CAD build for the part. Positions are in the model's coordinates, mm. A direction names the side the tool comes from. Give positions to 0.01 mm unless a question says otherwise; leave off trailing zeros. Order: outer loops, then holes, each group sorted by start corner. A loop starts at its lowest first (then second) coordinate and runs counter-clockwise, first axis right, second up.
Item 1: Band-saw the part on A-A on x = 0. Give the cut face in (y, z), plus the area to 3 significant figures.
Item 2: Band-saw the part on D-D on x = 4.5. Give the cut face in (y, z), plus the area to 3 significant figures.
Item 3: Two-plate mould, pull along Z, no slides. Class faces 1 (the cylindrical face through (14.14, 24.65, -14.1)), 2 (the flat face through (0, 50, -4)), 3 (the flat face through (-14, 25, -3.1)), 4 (the flat face through (-13.25, 25, 11)): released by +Z, released by -Z, zero draft, split by the parting line, or undercut.
Item 4: Band-saw the part on C-C on y = 17. Count the separate pieces of the cut face and the enclosed holes in it, plus the area to 3 significant figures.
Item 5: Wall check: L1, parallel to Z at x = -11, y = 19.5; L2, parallel to X at y = 24, z = 0; L3, parallel to X at y = 19, z = -6. Give the ranges that are in metal, low to high.
Item 6: Which spindle directions (+Z, -Z, +X, -X, +Y, -Y) get a long thin tool onto all of the face, cutting with end or side? Do faces 5 (the flat face through (-9.5, 25, -12)), 6 (the flat face through (15, 25, 8)). Say none if no direction does.
Item 7: Band-saw the part on B-B on z = 0. Give the cut face in (x, y).
Item 8: Flat gauge pins, fed straight in: P1, Ø6, axis at x = 11, z = -12, coming from the -Y side; P2, Ø1, axis at y = 19.5, z = 13, coming from the -X side; P3, Ø4.5, axis at x = 0, z = 0, coming from the +Y side; P4, Ø0.8, axis at y = 31.5, z = -13, coming from the -X side. Where does each tip first touch, or does it go through?
```python
from build123d import *

# Parameters (mm, degrees)
SKETCH2_R           = 2.5
BOSS_EXTRUDE1_DEPTH = 50


with BuildPart() as part:
    # Sketch2 → Boss-Extrude1 (new body)
    with BuildSketch(Plane(origin=(0, 0, 0), x_dir=(1, 0, 0), z_dir=(0, 1, 0))):
        with BuildLine():
            Line((3.6, -15), (12, -15))
            ThreePointArc((12, -15), (14.121320344, -14.121320344), (15, -12))
            Line((15, -12), (15, -3.6))
            ThreePointArc((15, -3.6), (14.853553391, -3.246446609), (14.5, -3.1))
            Line((14.5, -3.1), (12.5, -3.1))
            ThreePointArc((12.5, -3.1), (12.146446609, -3.246446609), (12, -3.6))
            Line((12, -3.6), (12, -5.6))
            Line((12, -5.6), (12.5, -5.6))
            ThreePointArc((12.5, -5.6), (12.853553391, -5.746446609), (13, -6.1))
            Line((13, -6.1), (13, -8.25))
            Line((13, -8.25), (10.492640687, -8.25))
            ThreePointArc((10.492640687, -8.25), (9.727273822, -8.097759065), (9.078427125, -7.664213562))
            Line((9.078427125, -7.664213562), (5.25, -3.835786438))
            Line((5.25, -3.835786438), (5.25, 3.835786438))
            Line((5.25, 3.835786438), (9.078427125, 7.664213562))
            ThreePointArc((9.078427125, 7.664213562), (9.727273822, 8.097759065), (10.492640687, 8.25))
            Line((10.492640687, 8.25), (13, 8.25))
            Line((13, 8.25), (13, 6.1))
            ThreePointArc((13, 6.1), (12.853553391, 5.746446609), (12.5, 5.6))
            Line((12.5, 5.6), (12, 5.6))
            Line((12, 5.6), (12, 3.6))
            ThreePointArc((12, 3.6), (12.146446609, 3.246446609), (12.5, 3.1))
            Line((12.5, 3.1), (14.5, 3.1))
            ThreePointArc((14.5, 3.1), (14.853553391, 3.246446609), (15, 3.6))
            Line((15, 3.6), (15, 12))
            ThreePointArc((15, 12), (14.121320344, 14.121320344), (12, 15))
            Line((12, 15), (-12, 15))
            ThreePointArc((-12, 15), (-14.121320344, 14.121320344), (-15, 12))
            Line((-15, 12), (-15, 3.6))
            ThreePointArc((-15, 3.6), (-14.853553391, 3.246446609), (-14.5, 3.1))
            Line((-14.5, 3.1), (-12.5, 3.1))
            ThreePointArc((-12.5, 3.1), (-12.146446609, 3.246446609), (-12, 3.6))
            Line((-12, 3.6), (-12, 5.6))
            Line((-12, 5.6), (-12.5, 5.6))
            ThreePointArc((-12.5, 5.6), (-12.853553391, 5.746446609), (-13, 6.1))
            Line((-13, 6.1), (-13, 8.25))
            Line((-13, 8.25), (-10.492640687, 8.25))
            ThreePointArc((-10.492640687, 8.25), (-9.727273822, 8.097759065), (-9.078427125, 7.664213562))
            Line((-9.078427125, 7.664213562), (-5.25, 3.835786438))
            Line((-5.25, 3.835786438), (-5.25, -3.835786438))
            Line((-5.25, -3.835786438), (-9.078427125, -7.664213562))
            ThreePointArc((-9.078427125, -7.664213562), (-9.727273822, -8.097759065), (-10.492640687, -8.25))
            Line((-10.492640687, -8.25), (-13, -8.25))
            Line((-13, -8.25), (-13, -6.1))
            ThreePointArc((-13, -6.1), (-12.853553391, -5.746446609), (-12.5, -5.6))
            Line((-12.5, -5.6), (-12, -5.6))
            Line((-12, -5.6), (-12, -3.6))
            ThreePointArc((-12, -3.6), (-12.146446609, -3.246446609), (-12.5, -3.1))
            Line((-12.5, -3.1), (-14.5, -3.1))
            ThreePointArc((-14.5, -3.1), (-14.853553391, -3.246446609), (-15, -3.6))
            Line((-15, -3.6), (-15, -12))
            ThreePointArc((-15, -12), (-14.121320344, -14.121320344), (-12, -15))
            Line((-12, -15), (-3.6, -15))
            ThreePointArc((-3.6, -15), (-3.246446609, -14.853553391), (-3.1, -14.5))
            Line((-3.1, -14.5), (-3.1, -12.5))
            ThreePointArc((-3.1, -12.5), (-3.246446609, -12.146446609), (-3.6, -12))
            Line((-3.6, -12), (-5.6, -12))
            Line((-5.6, -12), (-5.6, -12.5))
            ThreePointArc((-5.6, -12.5), (-5.746446609, -12.853553391), (-6.1, -13))
            Line((-6.1, -13), (-8, -13))
            Line((-8, -13), (-8, -10.242640687))
            ThreePointArc((-8, -10.242640687), (-7.847759065, -9.477273822), (-7.414213562, -8.828427125))
            Line((-7.414213562, -8.828427125), (-3.835786438, -5.25))
            Line((-3.835786438, -5.25), (3.835786438, -5.25))
            Line((3.835786438, -5.25), (7.414213562, -8.828427125))
            ThreePointArc((7.414213562, -8.828427125), (7.847759065, -9.477273822), (8, -10.242640687))
            Line((8, -10.242640687), (8, -13))
            Line((8, -13), (6.1, -13))
            ThreePointArc((6.1, -13), (5.746446609, -12.853553391), (5.6, -12.5))
            Line((5.6, -12.5), (5.6, -12))
            Line((5.6, -12), (3.6, -12))
            ThreePointArc((3.6, -12), (3.246446609, -12.146446609), (3.1, -12.5))
            Line((3.1, -12.5), (3.1, -14.5))
            ThreePointArc((3.1, -14.5), (3.246446609, -14.853553391), (3.6, -15))
        make_face()
        with Locations(Location((0, 0, 0), (0, 0, 270))):
            Circle(SKETCH2_R, mode=Mode.SUBTRACT)
        with BuildLine():
            Line((-3.835786438, 5.25), (3.835786438, 5.25))
            Line((3.835786438, 5.25), (7.414213562, 8.828427125))
            ThreePointArc((7.414213562, 8.828427125), (7.847759065, 9.477273822), (8, 10.242640687))
            Line((8, 10.242640687), (8, 13))
            Line((8, 13), (6.1, 13))
            ThreePointArc((6.1, 13), (5.746446609, 12.853553391), (5.6, 12.5))
            Line((5.6, 12.5), (5.6, 12))
            Line((5.6, 12), (3.6, 12))
            ThreePointArc((3.6, 12), (3.246446609, 12.146446609), (3.1, 12.5))
            Line((3.1, 12.5), (3.1, 14))
            Line((3.1, 14), (-3.1, 14))
            Line((-3.1, 14), (-3.1, 12.5))
            ThreePointArc((-3.1, 12.5), (-3.246446609, 12.146446609), (-3.6, 12))
            Line((-3.6, 12), (-5.6, 12))
            Line((-5.6, 12), (-5.6, 12.5))
            ThreePointArc((-5.6, 12.5), (-5.746446609, 12.853553391), (-6.1, 13))
            Line((-6.1, 13), (-8, 13))
            Line((-8, 13), (-8, 10.242640687))
            ThreePointArc((-8, 10.242640687), (-7.847759065, 9.477273822), (-7.414213562, 8.828427125))
            Line((-7.414213562, 8.828427125), (-3.835786438, 5.25))
        make_face(mode=Mode.SUBTRACT)
        with BuildLine():
            Line((9.5, -9.75), (13.25, -9.75))
            Line((13.25, -9.75), (13.25, -11.5))
            ThreePointArc((13.25, -11.5), (12.664213562, -12.914213562), (11.25, -13.5))
            Line((11.25, -13.5), (9.5, -13.5))
            Line((9.5, -13.5), (9.5, -9.75))
        make_face(mode=Mode.SUBTRACT)
        with BuildLine():
            Line((-13.25, -9.75), (-13.25, -11.5))
            ThreePointArc((-13.25, -11.5), (-12.664213562, -12.914213562), (-11.25, -13.5))
            Line((-11.25, -13.5), (-9.5, -13.5))
            Line((-9.5, -13.5), (-9.5, -9.75))
            Line((-9.5, -9.75), (-13.25, -9.75))
        make_face(mode=Mode.SUBTRACT)
        with BuildLine():
            Line((-9.5, 9.75), (-13.25, 9.75))
            Line((-13.25, 9.75), (-13.25, 11.5))
            ThreePointArc((-13.25, 11.5), (-12.664213562, 12.914213562), (-11.25, 13.5))
            Line((-11.25, 13.5), (-9.5, 13.5))
            Line((-9.5, 13.5), (-9.5, 9.75))
        make_face(mode=Mode.SUBTRACT)
        with BuildLine():
            Line((13.25, 9.75), (13.25, 11.5))
            ThreePointArc((13.25, 11.5), (12.664213562, 12.914213562), (11.25, 13.5))
            Line((11.25, 13.5), (9.5, 13.5))
            Line((9.5, 13.5), (9.5, 9.75))
            Line((9.5, 9.75), (13.25, 9.75))
        make_face(mode=Mode.SUBTRACT)
    extrude(amount=BOSS_EXTRUDE1_DEPTH)


solid = part.part
```
The answers:
1. outline: (0, -15) - (50, -15) - (50, -14) - (0, -14) - close; (0, -5.25) - (50, -5.25) - (50, -2.5) - (0, -2.5) - close; (0, 2.5) - (50, 2.5) - (50, 5.25) - (0, 5.25) - close
1. area: 325 mm2
2. outline: (0, -15) - (50, -15) - (50, -12) - (0, -12) - close; (0, -5.91) - (50, -5.91) - (50, 5.91) - (0, 5.91) - close; (0, 12) - (50, 12) - (50, 15) - (0, 15) - close
2. area: 891 mm2
3. face 1: released by -Z
3. face 2: zero draft
3. face 3: undercut
3. face 4: undercut
4. separate pieces: 1
4. enclosed holes: 6
4. area: 367 mm2
5. L1: z = -15 to -13.5, -9.75 to -8.25, 8.25 to 9.75, 13.5 to 15
5. L2: x = -5.25 to -2.5, 2.5 to 5.25
5. L3: x = -15 to -12.99, -7.41 to -4.59, 4.59 to 7.41, 12.99 to 15
6. face 5: +Y, -Y
6. face 6: +Z, -Z, +X, +Y, -Y
7. outline: (-5.25, 0) - (-2.5, 0) - (-2.5, 50) - (-5.25, 50) - close; (2.5, 0) - (5.25, 0) - (5.25, 50) - (2.5, 50) - close
8. P1: stops at y = 0
8. P2: stops at x = -14.96
8. P3: passes through
8. P4: stops at x = -14.94
